from build123d import *
from build123d import SkipClean  # not in build123d's __all__

# Parameters (mm, degrees)
F0_R     = 1.25
F0_R_2   = 4.5
F1_DEPTH = 20
F3_DEPTH = 19
F4_R     = 13.5
F4_R_2   = 10.5
F5_DEPTH = 3


with BuildPart() as f1:
    # F0 (on Top) → F1 (new body)
    with BuildSketch(Plane.XY):
        with BuildLine():
            Line((-10.5, 0), (-13.416407865, -1.5))
            ThreePointArc((-13.416407865, -1.5), (-9.545941546, -9.545941546), (-1.5, -13.416407865))
            Line((-1.5, -13.416407865), (0, -10.5))
            Line((0, -10.5), (1.5, -13.416407865))
            ThreePointArc((1.5, -13.416407865), (9.545941546, -9.545941546), (13.416407865, -1.5))
            Line((13.416407865, -1.5), (10.5, 0))
            Line((10.5, 0), (13.416407865, 1.5))
            ThreePointArc((13.416407865, 1.5), (9.545941546, 9.545941546), (1.5, 13.416407865))
            Line((1.5, 13.416407865), (0, 10.5))
            Line((0, 10.5), (-1.5, 13.416407865))
            ThreePointArc((-1.5, 13.416407865), (-9.545941546, 9.545941546), (-13.416407865, 1.5))
            Line((-13.416407865, 1.5), (-10.5, 0))
        make_face()
        with Locations((-5.6568542495, -5.6568542495)):
            Circle(F0_R, mode=Mode.SUBTRACT)
        with Locations((0, -8)):
            Circle(F0_R, mode=Mode.SUBTRACT)
        with Locations((5.6568542495, -5.6568542495)):
            Circle(F0_R, mode=Mode.SUBTRACT)
        with Locations((-8, 0)):
            Circle(F0_R, mode=Mode.SUBTRACT)
        with Locations((-5.6568542495, 5.6568542495)):
            Circle(F0_R, mode=Mode.SUBTRACT)
        Circle(F0_R_2, mode=Mode.SUBTRACT)
        with Locations((5.6568542495, 5.6568542495)):
            Circle(F0_R, mode=Mode.SUBTRACT)
        with Locations((8, 0)):
            Circle(F0_R, mode=Mode.SUBTRACT)
        with Locations((0, 8)):
            Circle(F0_R, mode=Mode.SUBTRACT)
    extrude(amount=F1_DEPTH)

    # F2 (on face) → F3 (cut)
    with BuildSketch(Plane.XY.offset(20)):
        with BuildLine():
            ThreePointArc((-7.0083017238, 3.8579407652), (-7.3910362601, 3.0614674589), (-7.68359375, 2.2276415971))
            ThreePointArc((-7.68359375, 2.2276415971), (-10.25, 0), (-7.68359375, -2.2276415971))
            ThreePointArc((-7.68359375, -2.2276415971), (-7.3910362601, -3.0614674589), (-7.0083017238, -3.8579407652))
            ThreePointArc((-7.0083017238, -3.8579407652), (-7.2478445072, -7.2478445072), (-3.8579407652, -7.0083017238))
            ThreePointArc((-3.8579407652, -7.0083017238), (-3.0614674589, -7.3910362601), (-2.2276415971, -7.68359375))
            ThreePointArc((-2.2276415971, -7.68359375), (0, -10.25), (2.2276415971, -7.68359375))
            ThreePointArc((2.2276415971, -7.68359375), (3.0614674589, -7.3910362601), (3.8579407652, -7.0083017238))
            ThreePointArc((3.8579407652, -7.0083017238), (7.2478445072, -7.2478445072), (7.0083017238, -3.8579407652))
            ThreePointArc((7.0083017238, -3.8579407652), (7.3910362601, -3.0614674589), (7.68359375, -2.2276415971))
            ThreePointArc((7.68359375, -2.2276415971), (10.25, 0), (7.68359375, 2.2276415971))
            ThreePointArc((7.68359375, 2.2276415971), (7.3910362601, 3.0614674589), (7.0083017238, 3.8579407652))
            ThreePointArc((7.0083017238, 3.8579407652), (7.2478445072, 7.2478445072), (3.8579407652, 7.0083017238))
            ThreePointArc((3.8579407652, 7.0083017238), (3.0614674589, 7.3910362601), (2.2276415971, 7.68359375))
            ThreePointArc((2.2276415971, 7.68359375), (0, 10.25), (-2.2276415971, 7.68359375))
            ThreePointArc((-2.2276415971, 7.68359375), (-3.0614674589, 7.3910362601), (-3.8579407652, 7.0083017238))
            ThreePointArc((-3.8579407652, 7.0083017238), (-7.2478445072, 7.2478445072), (-7.0083017238, 3.8579407652))
        make_face()
    extrude(amount=-F3_DEPTH, mode=Mode.SUBTRACT)

    # F4 (on face) → F5 (join)
    with BuildSketch(Plane(origin=(0, 0, 0), x_dir=(1, 0, 0), z_dir=(0, 0, -1))):
        Circle(F4_R)
        Circle(F4_R_2, mode=Mode.SUBTRACT)
    with SkipClean():  # cleaning this boolean's faces spoils the solid; the shape is the same uncleaned
        extrude(amount=-F5_DEPTH)


solid = f1.part
For this review, take the finished solid that the model builds, in its own axes (mm). A direction names the side the tool comes from. Coordinates: 2 decimals unless noted, no trailing zeros. Loops run counter-clockwise (first coordinate to the right, second up) from the corner with the lowest first, then second, coordinate; pieces in that order, holes last. Notation, with made-up numbers: (79, -30) - (134, -30) arc R21 ccw to (134, 7) - close; hole circle Ø11 at (-15, 3). An arc over 180 degrees is marked (long way). Return JSON: item names as keys, results as strings.
Item 1: Take a section at D-D (x = 8.5). Give the boundary of the cut face in (y, z).
Determined:
{"outline": "(-10.49, 0) - (-1.15, 0) - (-1.15, 1) - (-2.19, 1) - (-2.19, 20) - (-10.49, 20) - close; (1.15, 0) - (10.49, 0) - (10.49, 20) - (2.19, 20) - (2.19, 1) - (1.15, 1) - close"}
Item 2: For faces 3 (the cylindrical face through (-10.25, 0.05, 10.63)), 4 (the flat face through (11.94, 0.74, 11.38)), 5 (the flat face through (-11.98, 0.76, 11.38)), list the 3-axis set-ups (+Z, -Z, +X, -X, +Y, -Y) from which the entire face can be reached by the end or side of a thin tool; tool diameter is ignored.
Determined:
{"face 3": "+Z", "face 4": "+Z, +X", "face 5": "+Z, -X"}
Item 3: Take a section at B-B (x = -5). Give the boundary of the cut face in (y, z).
Determined:
{"outline": "(-12.54, 0) - (-6.72, 0) - (-6.72, 1) - (-7.81, 1) - (-7.81, 20) - (-12.54, 20) - close; (-4.59, 0) - (4.59, 0) - (4.59, 1) - (-4.59, 1) - close; (6.72, 0) - (12.54, 0) - (12.54, 20) - (7.81, 20) - (7.81, 1) - (6.72, 1) - close"}
Item 4: For line 1 (Y direction, x = -7.25, z = 19); line 2 (Z direction, x = 5.5, y = 3.5); line 3 (X direction, y = -0.25, z = 1.75), list the stretches that pass through material, from the lowest coordinate up.
Determined:
{"line 1": "y = -11.39 to -7.25, -4.07 to -3.38, 3.38 to 4.07, 7.25 to 11.39", "line 2": "z = 0 to 1", "line 3": "x = -13.5 to -10.24, 10.24 to 13.5"}
Item 5: Take a section at C-C (y = -3). Give the boundary of the cut face in (x, z), then the cut area to 3 significant figures.
Determined:
{"outline": "(-13.16, 0) - (-3.35, 0) - (-3.35, 1) - (-7.42, 1) - (-7.42, 20) - (-13.16, 20) - close; (3.35, 0) - (13.16, 0) - (13.16, 20) - (7.42, 20) - (7.42, 1) - (3.35, 1) - close", "area": "238 mm2"}
Item 6: Insertion check: pin 1 (2 mm diameter, centred on y = -2, z = 5, fed in from +X); pin 2 (6 mm diameter, centred on x = -2.5, y = -3, fed in from +Z); pin 3 (3 mm diameter, centred on x = -4, z = 3, fed in from +Y). Each pin has a flat end and moves straight along its axis. Give the tip position at first contact, or say it passes through.
Determined:
{"pin 1": "stops at x = 13.42", "pin 2": "stops at z = 1", "pin 3": "stops at y = 13.27"}
Item 7: Mouldability with a two-part tool opening along Y and no side actions: class faces 1 (the flat face through (-0.74, 11.94, 11.38)), 2 (the flat face through (-5, 0, 1)) as pulls with the +Y half, pulls with the -Y half, needs draft (parallel to the pull), parting line crosses it, or undercut.
Determined:
{"face 1": "pulls with the +Y half", "face 2": "undercut"}
Item 8: Take a section at A-A (z = 9.25). Give the boundary of the cut face in (x, y), then the cut area to 3 significant figures.
Determined:
{"outline": "(-13.42, -1.5) arc R13.5 ccw to (-1.5, -13.42) - (0, -10.5) - (1.5, -13.42) arc R13.5 ccw to (13.42, -1.5) - (10.5, 0) - (13.42, 1.5) arc R13.5 ccw to (1.5, 13.42) - (0, 10.5) - (-1.5, 13.42) arc R13.5 ccw to (-13.42, 1.5) - (-10.5, 0) - close; hole (-7.68, -2.23) arc R8 ccw to (-7.01, -3.86) arc R2.25 ccw (long way) to (-3.86, -7.01) arc R8 ccw to (-2.23, -7.68) arc R2.25 ccw (long way) to (2.23, -7.68) arc R8 ccw to (3.86, -7.01) arc R2.25 ccw (long way) to (7.01, -3.86) arc R8 ccw to (7.68, -2.23) arc R2.25 ccw (long way) to (7.68, 2.23) arc R8 ccw to (7.01, 3.86) arc R2.25 ccw (long way) to (3.86, 7.01) arc R8 ccw to (2.23, 7.68) arc R2.25 ccw (long way) to (-2.23, 7.68) arc R8 ccw to (-3.86, 7.01) arc R2.25 ccw (long way) to (-7.01, 3.86) arc R8 ccw to (-7.68, 2.23) arc R2.25 ccw (long way) to start", "area": "286 mm2"}
